```python
from build123d import *

# Parameters (mm, degrees)
F1_DEPTH = 12
F2_R     = 5
F3_R     = 2
F4_DEPTH = 69.001
F5_R     = 4
F6_R     = 2
F7_DEPTH = 12
F8_R     = 1.5
F9_DEPTH = 25
F10_R    = 1


with BuildPart() as f1:
    # F0 (on Top) → F1 (new body)
    with BuildSketch(Plane.XY):
        with BuildLine():
            Line((52.5, 0), (-52.5, 0))
            Line((-52.5, 0), (-46.6771353676, -15.9990389547))
            ThreePointArc((-46.6771353676, -15.9990389547), (-44.7400164437, -19.1834804046), (-41.7268534535, -21.3775510204))
            ThreePointArc((-41.7268534535, -21.3775510204), (-36.0124674438, -25.9915106654), (-33.1735048367, -32.7652188367))
            Line((-33.1735048367, -32.7652188367), (-31.7911865206, -41.93988096))
            ThreePointArc((-31.7911865206, -41.93988096), (-27.6690936208, -53.5220419681), (-19.5011770908, -62.7102541473))
            Line((-19.5011770908, -62.7102541473), (-16.5, -65))
            Line((-16.5, -65), (-16.5, -80))
            Line((-16.5, -80), (-1.5, -80))
            Line((-1.5, -80), (-1.5, -59.2491515674))
            ThreePointArc((-1.5, -59.2491515674), (0, -15), (1.5, -59.2491515674))
            Line((1.5, -59.2491515674), (1.5, -80))
            Line((1.5, -80), (16.5, -80))
            Line((16.5, -80), (16.5, -65))
            Line((16.5, -65), (19.5011770908, -62.7102541473))
            ThreePointArc((19.5011770908, -62.7102541473), (27.6690936208, -53.5220419681), (31.7911865206, -41.93988096))
            Line((31.7911865206, -41.93988096), (33.1735048367, -32.7652188367))
            ThreePointArc((33.1735048367, -32.7652188367), (36.0124674438, -25.9915106654), (41.7268534535, -21.3775510204))
            ThreePointArc((41.7268534535, -21.3775510204), (44.7400164437, -19.1834804046), (46.6771353676, -15.9990389547))
            Line((46.6771353676, -15.9990389547), (52.5, 0))
        make_face()
        with BuildLine():
            Line((-34.25, -15.5), (-37.75, -15.5))
            ThreePointArc((-37.75, -15.5), (-40.5, -12.75), (-37.75, -10))
            Line((-37.75, -10), (-34.25, -10))
            ThreePointArc((-34.25, -10), (-31.5, -12.75), (-34.25, -15.5))
        make_face(mode=Mode.SUBTRACT)
        with BuildLine():
            ThreePointArc((37.75, -10), (40.5, -12.75), (37.75, -15.5))
            Line((37.75, -15.5), (34.25, -15.5))
            ThreePointArc((34.25, -15.5), (31.5, -12.75), (34.25, -10))
            Line((34.25, -10), (37.75, -10))
        make_face(mode=Mode.SUBTRACT)
    extrude(amount=F1_DEPTH)

    # F2
    f2_edges = [f1.edges().sort_by_distance(p)[0] for p in [
        (-16.5, -65, 6),
        (16.5, -65, 6),
    ]]
    fillet(f2_edges, radius=F2_R)

    # F3 (on face) → F4 (cut, through all)
    with BuildSketch(Plane(origin=(-16.5, 0, 0), x_dir=(0, -1, 0), z_dir=(-1, 0, 0))):
        with Locations((72.5, 6)):
            Circle(F3_R)
    extrude(amount=-F4_DEPTH, mode=Mode.SUBTRACT)

    # F5
    f5_edges = [f1.edges().sort_by_distance(p)[0] for p in [
        (-16.5, -80, 6),
        (16.5, -80, 6),
    ]]
    fillet(f5_edges, radius=F5_R)

    # F6 (on face) → F7 (cut)
    with BuildSketch(Plane(origin=(0, 0, 0), x_dir=(-1, 0, 0), z_dir=(0, 1, 0))):
        with Locations((-36, 6)):
            Circle(F6_R)
        with Locations((36, 6)):
            Circle(F6_R)
    extrude(amount=-F7_DEPTH, mode=Mode.SUBTRACT)

    # F8 (on face) → F9 (cut)
    with BuildSketch(Plane.XY.offset(12)):
        with Locations((0, -15)):
            Circle(F8_R)
        with Locations((-19.1824626938, -48.225)):
            Circle(F8_R)
        with Locations((19.1824626938, -48.225)):
            Circle(F8_R)
    extrude(amount=-F9_DEPTH, mode=Mode.SUBTRACT)

    # F10
    f10_edges = [f1.edges().sort_by_distance(p)[0] for p in [
        (1.49914, -15.05079, 6),
        (-1.49914, -15.05079, 6),
        (-19.888047, -46.901312, 6),
        (-18.388907, -49.497898, 6),
        (18.388907, -49.497898, 6),
        (19.888047, -46.901312, 6),
        (1.5, -59.249152, 6),
        (-1.5, -59.249152, 6),
        (1.5, -80, 6),
        (-1.5, -80, 6),
    ]]
    fillet(f10_edges, radius=F10_R)


solid = f1.part
```
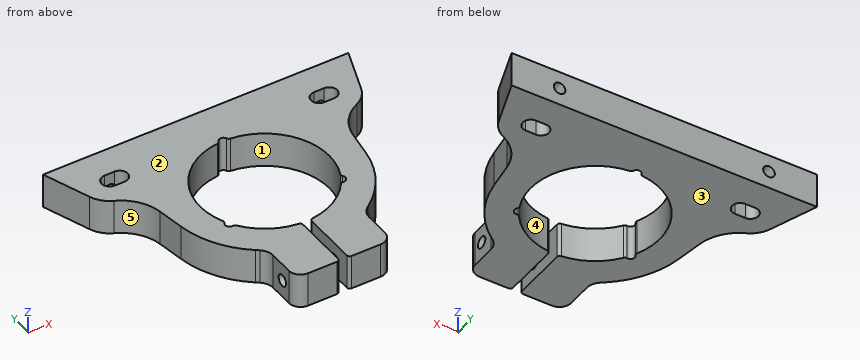
Source: CAD feature listing. Evaluate the final solid. Frame: model axes, mm. Face numbers are marked on the shaded views. A direction names the side the tool comes from. Round coordinates to 2 decimals unless told otherwise and drop trailing zeros. Write each loop counter-clockwise with the first axis right and the second up, starting at its lowest first coordinate (ties: lowest second). Pieces come first, ordered by that corner, then holes. Notation, with made-up numbers: M 44,2.25 L 94,2.25 A21 cw 94,22.25 Z; hole C 13.5,62.25 d3. An arc over 180 degrees is marked long. Answer as a JSON object with one key per item and string values. Group by question number.
(1) Mould query, pull axis X, two halves, no side actions, for the marked faces 3, 4 and 5. Classes: +X half, -X half, draft (parallel to the pull), parting line (faces both ways), or undercut.
(2) First-contact query: pin 1 (1 mm diameter, centred on x = -35.5, z = 2.5, fed in from -Y); pin 2 (1.5 mm diameter, centred on y = -27, z = 4.5, fed in from -X); pin 3 (2.5 mm diameter, centred on y = -72, z = 8.5, fed in from -X); pin 4 (2 mm diameter, centred on x = 25, z = 5.5, fed in from +Y). Flat tips, straight axial feed; report the tip coordinate or a pass-through.
(3) Section query A-A on y = -72.5. Output: boundary loops of the cut face in (x, z), then the cut area to 3 significant figures.
(4) Section query B-B on x = 36. Output: boundary loops of the cut face in (y, z), then the cut area to 3 significant figures.
(5) Section query D-D on z = 9.75. State how many separate pieces and enclosed holes the cut face has, then the cut area to 3 significant figures.
(6) Section query C-C on y = -44.5. Output: boundary loops of the cut face in (x, z), then the cut area to 3 significant figures.
(7) Reachability of the marked faces 1 and 2 from +Z, -Z, +X, -X, +Y, -Y: full face, straight path, thin tool, end or side. Return the list, or none.
(8) Ray query, line 1 (X direction, y = -10.5, z = 8.5); line 2 (X direction, y = -68, z = 6.5); line 3 (X direction, y = -14, z = 11). Return the intervals inside material, ascending. Write a range as [from, to].
Computed values:
{
 "1": {"face 3": "draft", "face 4": "undercut", "face 5": "-X half"},
 "2": {"pin 1": "y = -27.53", "pin 2": "x = -35.82", "pin 3": "x = -16.5", "pin 4": "y = 0"},
 "3": {"outline": "M -16.5,0 L -1.5,0 L -1.5,4 L -16.5,4 Z; M -16.5,8 L -1.5,8 L -1.5,12 L -16.5,12 Z; M 1.5,0 L 16.5,0 L 16.5,4 L 1.5,4 Z; M 1.5,8 L 16.5,8 L 16.5,12 L 1.5,12 Z", "area": "240 mm^2"},
 "4": {"outline": "M -26.01,0 L -15.5,0 L -15.5,12 L -26.01,12 Z; M -10,0 L 0,0 L 0,4 L -10,4 Z; M -10,8 L 0,8 L 0,12 L -10,12 Z", "area": "206 mm^2"},
 "5": {"separate pieces": "1", "enclosed holes": "2", "area": "3,500 mm^2"},
 "6": {"outline": "M -31.3,0 L -20.89,0 L -20.89,12 L -31.3,12 Z; M 20.89,0 L 31.3,0 L 31.3,12 L 20.89,12 Z", "area": "250 mm^2"},
 "7": {"face 1": "+Z, -Z", "face 2": "+Z, +X, -X, +Y, -Y"},
 "8": {"line 1": "[-48.68, -39.33], [-32.67, 32.67], [39.33, 48.68]", "line 2": "[-16.5, -1.5], [1.5, 16.5]", "line 3": "[-47.4, -40.2], [-31.8, -1.12], [1.12, 31.8], [40.2, 47.4]"}
}
